CAD build for the part. Positions are in the model's coordinates, mm. Give positions to 0.01 mm unless a question says otherwise; leave off trailing zeros. Write each loop counter-clockwise with the first axis right and the second up, starting at its lowest first coordinate (ties: lowest second). Pieces come first, ordered by that corner, then holes. Notation, with made-up numbers: (18.5, 18.5) -> (70.5, 18.5) arc R14 cw to (70.5, 25.5) -> close; hole circle Ø3 at (-5, 5). An arc over 180 degrees is marked (long way). Answer as a JSON object with one key per item and string values.
```python
from build123d import *

# Parameters (mm, degrees)
F1_DEPTH = 2.5
F2_W     = 5
F2_H     = 10
F2_W_2   = 10
F2_H_2   = 5
F3_DEPTH = 5
F4_SIZE  = 4


with BuildPart() as f1:
    # F0 (on Front) → F1 (new body, symmetric)
    with BuildSketch(Plane.XZ):
        Polygon((-30, -30), (30, -30), (30, -15), (-15, 30), (-30, 30), align=None)
    extrude(amount=F1_DEPTH, both=True)

    # F2 (on face) → F3 (join, through all)
    with BuildSketch(Plane.XZ.offset(2.5)):
        with Locations((-32.5, 25)):
            Rectangle(F2_W, F2_H)
        with Locations((-32.5, 5)):
            Rectangle(F2_W, F2_H)
        with Locations((-32.5, -15)):
            Rectangle(F2_W, F2_H)
        with Locations((25, -32.5)):
            Rectangle(F2_W_2, F2_H_2)
        with Locations((5, -32.5)):
            Rectangle(F2_W_2, F2_H_2)
        with Locations((-15, -32.5)):
            Rectangle(F2_W_2, F2_H_2)
    extrude(amount=-F3_DEPTH)

    # F4
    f4_edges = [f1.edges().sort_by_distance(p)[0] for p in [
        (-30, 0, -30),
    ]]
    chamfer(f4_edges, length=F4_SIZE)


solid = f1.part
```
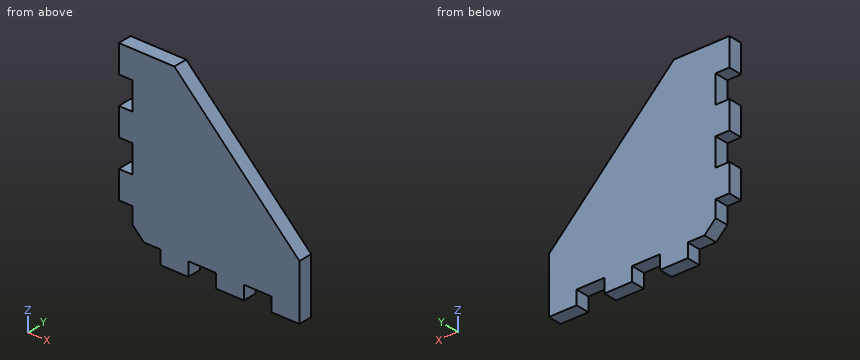
1) Slice it at A-A (y = 1.15). List the corners of the cut face in (x, z), then the cut area to 3 significant figures.
Model answer:
{"outline": "(-35, -20) -> (-30, -20) -> (-30, -26) -> (-26, -30) -> (-20, -30) -> (-20, -35) -> (-10, -35) -> (-10, -30) -> (0, -30) -> (0, -35) -> (10, -35) -> (10, -30) -> (20, -30) -> (20, -35) -> (30, -35) -> (30, -15) -> (-15, 30) -> (-35, 30) -> (-35, 20) -> (-30, 20) -> (-30, 10) -> (-35, 10) -> (-35, 0) -> (-30, 0) -> (-30, -10) -> (-35, -10) -> close", "area": "2,880 mm2"}
2) Pin check, flat tips, straight feed: pin 1 (1.5 mm diameter, centred on y = -0.5, z = -32, fed in from -X); pin 2 (2 mm diameter, centred on x = 19.5, y = -0.5, fed in from +Z); pin 3 (2.5 mm diameter, centred on y = -0.5, z = -6, fed in from -X). Stop position of each tip, or through.
Model answer:
{"pin 1": "stops at x = -20", "pin 2": "stops at z = -3.5", "pin 3": "stops at x = -30"}
3) Slice it at B-B (z = 25). List the corners of the cut face in (x, y).
Model answer:
{"outline": "(-35, -2.5) -> (-10, -2.5) -> (-10, 2.5) -> (-35, 2.5) -> close"}
4) Wall check: probe 1 along X at (y, z) = (1.55, -31.5); probe 2 along Z at (x, y) = (-26, -0.85). Give the ranges that are in metal, low to high.
Model answer:
{"probe 1": "x = -20 to -10, 0 to 10, 20 to 30", "probe 2": "z = -30 to 30"}
5) Slice it at C-C (x = 26). List the corners of the cut face in (y, z), then the cut area to 3 significant figures.
Model answer:
{"outline": "(-2.5, -35) -> (2.5, -35) -> (2.5, -11) -> (-2.5, -11) -> close", "area": "120 mm2"}
